Design review of the part built by this model. Coordinates are the model's own, in mm. A direction names the side the tool comes from. Give positions to 0.01 mm unless a question says otherwise; leave off trailing zeros. Loops run counter-clockwise (first coordinate to the right, second up) from the corner with the lowest first, then second, coordinate; pieces in that order, holes last. Notation, with made-up numbers: M -28,2.5 L 27,2.5 A23 ccw 27,10.5 Z; hole C 43.25,23.25 d3. An arc over 180 degrees is marked long. Answer as CSV lines item,"result".
```python
from build123d import *

# Parameters (mm, degrees)
BASE_FLANGE1_DEPTH  = 2.5
SKETCH6_W           = 0.4
SKETCH6_H           = 3.67
BOSS_EXTRUDE1_DEPTH = 4.5
SKETCH7_W           = 3.4
SKETCH7_H           = 1
CUT_EXTRUDE1_DEPTH  = 4.5
FILLET1_RADIUS      = 1.335
FILLET1_LENGTH      = 0.4


# Sheet-metal steps are written as plain solids
with BuildPart() as part:
    # Sketch1 → Base-Flange1 (new body)
    with BuildSketch(Plane.XY):
        with BuildLine():
            Line((0.71, 0), (0.71, 3.67))
            ThreePointArc((0.71, 3.67), (0, 4.38), (-0.71, 3.67))
            Line((-0.71, 3.67), (-0.71, -0.5))
            ThreePointArc((-0.71, -0.5), (-0.998929703, -1.045808423), (-1.612747985, -1.113737253))
            Line((-1.612747985, -1.113737253), (-6.727225094, 0.909162621))
            Line((-6.727225094, 0.909162621), (-6.580105103, 1.281124592))
            Line((-6.580105103, 1.281124592), (-1.465627994, -0.741775282))
            ThreePointArc((-1.465627994, -0.741775282), (-1.223820792, -0.71501544), (-1.11, -0.5))
            Line((-1.11, -0.5), (-1.11, 3.67))
            ThreePointArc((-1.11, 3.67), (0, 4.78), (1.11, 3.67))
            Line((1.11, 3.67), (1.11, 0))
            Line((1.11, 0), (0.71, 0))
        make_face()
    extrude(amount=BASE_FLANGE1_DEPTH)

    # Sketch6 → Boss-Extrude1 (add)
    with BuildSketch(Plane.XY.offset(2.5)):
        with Locations((0.91, 1.835)):
            Rectangle(SKETCH6_W, SKETCH6_H)
    extrude(amount=BOSS_EXTRUDE1_DEPTH)

    # Sketch7 → Cut-Extrude1 (cut)
    with BuildSketch(Plane(origin=(1.11, 0, 0), x_dir=(0, 0, -1), z_dir=(1, 0, 0))):
        with Locations((-5.3, 0.5)):
            Rectangle(SKETCH7_W, SKETCH7_H)
    extrude(amount=-CUT_EXTRUDE1_DEPTH, mode=Mode.SUBTRACT)

    # Fillet1: full round fillet: the end face becomes a half cylinder, R = half its width
    fillet1_face = Plane((0.91, 2.335, 7), x_dir=(-1, 0, 0), z_dir=(0, 0, 1))  # on the end face: x along it, z out of the body
    fillet1_slab = fillet1_face.offset(-FILLET1_RADIUS / 2) * Box(FILLET1_LENGTH, 2 * FILLET1_RADIUS, FILLET1_RADIUS, mode=Mode.PRIVATE)  # the body's end, R deep
    fillet1_round = Plane((0.91, 2.335, 5.665), x_dir=(0, 0, 1), z_dir=(-1, 0, 0)) * Cylinder(FILLET1_RADIUS, FILLET1_LENGTH, mode=Mode.PRIVATE)  # its axis R under the face
    add(fillet1_slab - fillet1_round, mode=Mode.SUBTRACT)


solid = part.part
```
1. We need section A-A, the plane z = 1. Write out the cut boundary in (x, y), plus the area to 3 significant figures.
Answer block:
outline,"M -6.73,0.91 L -1.61,-1.11 A0.66 ccw -0.71,-0.5 L -0.71,3.67 A0.71 cw 0.71,3.67 L 0.71,0 L 1.11,0 L 1.11,3.67 A1.11 ccw -1.11,3.67 L -1.11,-0.5 A0.26 cw -1.47,-0.74 L -6.58,1.28 Z"
area,"6.84 mm²"
2. We need section D-D, the plane x = 0. Write out the cut boundary in (y, z), plus the area to 3 significant figures.
Answer block:
outline,"M 4.38,0 L 4.78,0 L 4.78,2.5 L 4.38,2.5 Z"
area,"1.00 mm²"
3. For faces 1 (the flat face through (1.11, 2, 3)), 2 (the flat face through (0.71, 2, 3)), 3 (the flat face through (-1.11, 2, 1)), list the 3-axis set-ups (+Z, -Z, +X, -X, +Y, -Y) from which the entire face can be reached by the end or side of a thin tool; tool diameter is ignored.
Answer block:
face 1,"+Z, -Z, +X, +Y, -Y"
face 2,"+Z, -Z, -Y"
face 3,"+Z, -Z, +Y"
4. For P1, Ø2, axis at y = 0.5, z = 1.5, coming from the -X side, flat-tipped, find the tip position at first contact; note if it passes through.
Answer block:
P1,"x = -6.73"
5. We need section B-B, the plane y = 4.1. Write out the cut boundary in (x, z).
Answer block:
outline,"M -1.02,0 L -0.56,0 L -0.56,2.5 L -1.02,2.5 Z; M 0.56,0 L 1.02,0 L 1.02,2.5 L 0.56,2.5 Z"
6. To check wall thickness, follow L1, parallel to X at y = 1.65, z = 4.25; L2, parallel to Z at x = -1, y = 3.85; L3, parallel to Y at x = 0.75, z = 1.75. State the ranges of each line that lie inside material, in increasing order. Write a range as [from, to].
Answer block:
L1,"[0.71, 1.11]"
L2,"[0, 2.5]"
L3,"[0, 4.49]"
7. We need section C-C, the plane y = 0.45. Write out the cut boundary in (x, z), plus the area to 3 significant figures.
Answer block:
outline,"M -5.57,0 L -4.48,0 L -4.48,2.5 L -5.57,2.5 Z; M -1.11,0 L -0.71,0 L -0.71,2.5 L -1.11,2.5 Z; M 0.71,0 L 1.11,0 L 1.11,3.6 L 0.71,3.6 Z"
area,"5.16 mm²"
